Here's how the part is built. I have some questions about the finished solid (model axes, mm). A direction names the side the tool comes from. Round coordinates to 2 decimals unless told otherwise and drop trailing zeros. Write each loop counter-clockwise with the first axis right and the second up, starting at its lowest first coordinate (ties: lowest second). Pieces come first, ordered by that corner, then holes. Notation, with made-up numbers: (24, 25.5) -> (69, 25.5) arc R14 ccw to (69, 30.5) -> close; hole circle Ø11 at (58, 46). An arc over 180 degrees is marked (long way). Put each result on its own line as item: value. Start each with the question number.
1) Will these pins go through, and if not, where does the flat tip stop? P1, Ø4, axis at x = -19.5, z = 11, coming from the -Y side; P2, Ø5, axis at x = 13.5, z = 11.5, coming from the -Y side; P3, Ø4, axis at x = 15, z = 8.5, coming from the +Y side.
2) I want a section at A-A, the plane z = 1. Give the number of separate pieces and of enclosed holes in the cut face, then the cut area to 3 significant figures.
3) If I drill on line 1 along Y through (x, z) = (-11, 5.25); line 2 along Y through (x, z) = (18, 8.25); line 3 along Z through (x, y) = (15.5, -14), over which ranges is the centre line in solid material (lowest first)? Write a range as [from, to].
4) I want a section at B-B, the plane y = -5.5. List the corners of the cut face in (x, z) for me.
5) Which directions (+Z, -Z, +X, -X, +Y, -Y) give clear straight access to the entire face, cutting with the end or side of a thin tool? Please do faces 1 (the flat face through (0, 17, 0)), 2 (the flat face through (-8.063, 2.326, 5.07)).
6) We'd pull the mould along Y, two halves only. Please class faces 3 (the flat face through (-17, 0, 0)), 4 (the flat face through (-2.326, -8.063, 5.07)): released by +Y, released by -Y, zero draft, split by the parting line, or undercut.
7) I want a section at D-D, the plane y = 12. List the corners of the cut face in (x, z) for me.
8) I want a section at C-C, the plane x = 20.5. List the corners of the cut face in (y, z) for me.
from build123d import *

# Parameters (mm, degrees)
F0_R     = 25
F1_DEPTH = 15
F2_R     = 23.5
F3_DEPTH = 10
F6_DEPTH = 10
F7_DEPTH = 10


with BuildPart() as f1:
    # F0 (on Top) → F1 (new body)
    with BuildSketch(Plane.XY):
        Circle(F0_R)
    extrude(amount=F1_DEPTH)

    # F2 (on face) → F3 (cut)
    with BuildSketch(Plane(origin=(0, 0, 0), x_dir=(1, 0, 0), z_dir=(0, 0, -1))):
        Circle(F2_R)
    extrude(amount=-F3_DEPTH, mode=Mode.SUBTRACT)

    # F5 (on face) → F6 (join)
    with BuildSketch(Plane(origin=(0, 0, 10), x_dir=(1, 0, 0), z_dir=(0, 0, -1))):
        Polygon((0, -10.9), (4.5870057685, -9), (0, -7.1), (-4.5870057685, -9), align=None)
        Polygon((7.1, 0), (9, -4.5870057685), (10.9, 0), (9, 4.5870057685), align=None)
        Polygon((0, 7.1), (4.5870057685, 9), (0, 10.9), (-4.5870057685, 9), align=None)
        Polygon((-7.1, 0), (-9, 4.5870057685), (-10.9, 0), (-9, -4.5870057685), align=None)
        Polygon((0, 15.1), (4.5870057685, 17), (0, 18.9), (-4.5870057685, 17), align=None)
        Polygon((-15.2643181644, 8.7773123959), (-10.6773123959, 10.6773123959), (-8.7773123959, 15.2643181644), (-13.3643181644, 13.3643181644), align=None)
        Polygon((-17, -4.5870057685), (-15.1, 0), (-17, 4.5870057685), (-18.9, 0), align=None)
        Polygon((-8.7773123959, -15.2643181644), (-10.6773123959, -10.6773123959), (-15.2643181644, -8.7773123959), (-13.3643181644, -13.3643181644), align=None)
        Polygon((4.5870057685, -17), (0, -15.1), (-4.5870057685, -17), (0, -18.9), align=None)
        Polygon((15.2643181644, -8.7773123959), (10.6773123959, -10.6773123959), (8.7773123959, -15.2643181644), (13.3643181644, -13.3643181644), align=None)
        Polygon((17, 4.5870057685), (15.1, 0), (17, -4.5870057685), (18.9, 0), align=None)
        Polygon((8.7773123959, 15.2643181644), (10.6773123959, 10.6773123959), (15.2643181644, 8.7773123959), (13.3643181644, 13.3643181644), align=None)
    extrude(amount=F6_DEPTH)

    # F4 (on face) → F7 (join)
    with BuildSketch(Plane(origin=(0, 0, 10), x_dir=(1, 0, 0), z_dir=(0, 0, -1))):
        with BuildLine():
            add(Edge.make_bspline(
                [(0, 3), (0, 1.9449878018), (1.905477955, 0), (3, 0)],
                knots=[0, 0, 0, 0, 4.2426406871, 4.2426406871, 4.2426406871, 4.2426406871], degree=3))
            add(Edge.make_bspline(
                [(0, 3), (0, 1.9449878018), (-1.905477955, 0), (-3, 0)],
                knots=[0, 0, 0, 0, 4.2426406871, 4.2426406871, 4.2426406871, 4.2426406871], degree=3))
            add(Edge.make_bspline(
                [(0, -3), (0, -1.9449878018), (-1.905477955, 0), (-3, 0)],
                knots=[0, 0, 0, 0, 4.2426406871, 4.2426406871, 4.2426406871, 4.2426406871], degree=3))
            add(Edge.make_bspline(
                [(0, -3), (0, -1.9449878018), (1.905477955, 0), (3, 0)],
                knots=[0, 0, 0, 0, 4.2426406871, 4.2426406871, 4.2426406871, 4.2426406871], degree=3))
        make_face()
    extrude(amount=F7_DEPTH)


solid = f1.part
Findings:
1. P1: stops at y = -17.85
1. P2: stops at y = -22.45
1. P3: stops at y = 21.35
2. separate pieces: 14
2. enclosed holes: 1
2. area: 449 mm2
3. line 1: y = [-22.45, -20.77], [-14.34, -10.54], [10.54, 14.34], [20.77, 22.45]
3. line 2: y = [-17.35, -15.11], [-2.17, 2.17], [15.11, 17.35]
3. line 3: z = [10, 15]
4. outline: (-24.39, 0) -> (-22.85, 0) -> (-22.85, 10) -> (22.85, 10) -> (22.85, 0) -> (24.39, 0) -> (24.39, 15) -> (-24.39, 15) -> close
5. face 1: -Z, +X, -X, +Y, -Y
5. face 2: -Z
6. face 3: zero draft
6. face 4: undercut
7. outline: (-21.93, 0) -> (-20.21, 0) -> (-20.21, 10) -> (-13.93, 10) -> (-13.93, 0) -> (-10.13, 0) -> (-10.13, 10) -> (10.13, 10) -> (10.13, 0) -> (13.93, 0) -> (13.93, 10) -> (20.21, 10) -> (20.21, 0) -> (21.93, 0) -> (21.93, 15) -> (-21.93, 15) -> close
8. outline: (-14.31, 0) -> (-11.49, 0) -> (-11.49, 10) -> (11.49, 10) -> (11.49, 0) -> (14.31, 0) -> (14.31, 15) -> (-14.31, 15) -> close
